from build123d import *

# Parameters (mm, degrees)
EXTRUDE_1_DEPTH     = 22.5
SKETCH_2_R          = 11
CUT_EXTRUDE_2_DEPTH = 18
CUT_EXTRUDE_3_REACH = 24.5
SKETCH_3_R          = 4
CHAMFER_1_SIZE      = 1


with BuildPart() as part:
    # Эскиз1 → Бобышка-Вытянуть1 (new body)
    with BuildSketch(Plane(origin=(0, 0, 0), x_dir=(1, 0, 0), z_dir=(0, 1, 0))):
        Polygon((17.320508076, 0), (8.660254038, 15), (-8.660254038, 15), (-17.320508076, 0), (-8.660254038, -15), (8.660254038, -15), align=None)
    extrude(amount=EXTRUDE_1_DEPTH)

    # Эскиз2 → Вырез-Вытянуть2 (cut)
    with BuildSketch(Plane(origin=(0, 22.5, 0), x_dir=(1, 0, 0), z_dir=(0, 1, 0))):
        Circle(SKETCH_2_R)
    extrude(amount=-CUT_EXTRUDE_2_DEPTH, mode=Mode.SUBTRACT)

    # Эскиз3 → Вырез-Вытянуть3 (cut, up to next)
    with BuildSketch(Plane.XZ, mode=Mode.PRIVATE) as cut_extrude_3_sk1:
        Circle(SKETCH_3_R)
    cut_extrude_3_tool1 = extrude(cut_extrude_3_sk1.sketch, amount=-CUT_EXTRUDE_3_REACH, mode=Mode.PRIVATE) & part.part
    add(cut_extrude_3_tool1.solids().sort_by_distance((0, 0, 0))[0], mode=Mode.SUBTRACT)

    # Эскиз4 → Вырез-Повернуть1 (revolve, cut)
    with BuildSketch(Plane(origin=(0, 0, 0), x_dir=(-0.5, 0, 0.866025404), z_dir=(-0.866025404, 0, -0.5))):
        Polygon((-17.320508076, 18.345818937), (-17.320508076, 22.5), (-14.628303654, 22.5), align=None)
    cut_revolve_1 = revolve(axis=Axis((0, 0, 0), (0, 1, 0)), mode=Mode.SUBTRACT)

    # Зеркальное отражение1: Вырез-Повернуть1 across plane
    add(cut_revolve_1.mirror(Plane.ZX.offset(11.25)), mode=Mode.SUBTRACT)

    # Фаска1
    chamfer_1_edges = [part.edges().sort_by_distance(p)[0] for p in [
        (-11, 22.5, 0),
    ]]
    chamfer(chamfer_1_edges, length=CHAMFER_1_SIZE)


solid = part.part
Design review of the part built by this model. Coordinates are the model's own, in mm. A direction names the side the tool comes from. Coordinates: 2 decimals unless noted, no trailing zeros. Loops run counter-clockwise (first coordinate to the right, second up) from the corner with the lowest first, then second, coordinate; pieces in that order, holes last.
Item 1: Clearance check with flat-ended pins moving along their axes: pin 1 (10 mm diameter, centred on x = 6.5, z = -0.5, fed in from -Y); pin 2 (1.5 mm diameter, centred on y = 7.5, z = 5, fed in from -X); pin 3 (1 mm diameter, centred on y = 5, z = 6.5, fed in from -X); pin 4 (17.5 mm diameter, centred on x = 0, z = 0, fed in from +Y). State where each tip first meets the part, or that it passes through.
Completed:
pin 1: stops at y = 0
pin 2: stops at x = -14.87
pin 3: stops at x = -13.86
pin 4: stops at y = 4.5
Item 2: For faces 1 (the flat face through (0, 11, -15)), 2 (the flat face through (0, 4.5, 5)), list the 3-axis set-ups (+Z, -Z, +X, -X, +Y, -Y) from which the entire face can be reached by the end or side of a thin tool; tool diameter is ignored.
Completed:
face 1: -Z, +X, -X, +Y, -Y
face 2: +Y
Item 3: Add section B-B (y = 16.75). Write out the cut boundary in (x, z).
Completed:
outline: (-17.32, 0) - (-8.66, -15) - (8.66, -15) - (17.32, 0) - (8.66, 15) - (-8.66, 15) - close; hole circle Ø22 at (0, 0)
Item 4: Add section A-A (x = 0). Write out the cut boundary in (y, z).
Completed:
outline: (0, -14.63) - (0.57, -15) - (21.93, -15) - (22.5, -14.63) - (22.5, -12) - (21.5, -11) - (4.5, -11) - (4.5, -4) - (0, -4) - close; (0, 4) - (4.5, 4) - (4.5, 11) - (21.5, 11) - (22.5, 12) - (22.5, 14.63) - (21.93, 15) - (0.57, 15) - (0, 14.63) - close
Item 5: Wall thickness on L1, parallel to Z at x = 0, y = 2.65; L2, parallel to Z at x = 0, y = 11; L3, parallel to X at y = 10.75, z = -10: over which ranges is each line inside the solid? List them lowest first.
Completed:
L1: z = -15 to -4, 4 to 15
L2: z = -15 to -11, 11 to 15
L3: x = -11.55 to -4.58, 4.58 to 11.55
Item 6: Draft analysis for pull direction Z (two halves, no side actions). For faces 3 (the cylindrical face through (-0.867, 2.218, -3.905)), 4 (the cylindrical face through (-2.38, 13.12, 10.74)), 5 (the flat face through (13.05, 11.1, -7.4)), 6 (the flat face through (0, 11, 15)), state which applies: pulls with the +Z half, pulls with the -Z half, needs draft (parallel to the pull), parting line crosses it, or undercut.
Completed:
face 3: undercut
face 4: undercut
face 5: pulls with the -Z half
face 6: pulls with the +Z half
Item 7: Add section C-C (y = 19.75). Write out the cut boundary in (x, z).
Completed:
outline: (-16.32, -1.74) - (-9.66, -13.26) arc R16.41 ccw to (-6.66, -15) - (6.66, -15) arc R16.41 ccw to (9.66, -13.26) - (16.32, -1.74) arc R16.41 ccw to (16.32, 1.74) - (9.66, 13.26) arc R16.41 ccw to (6.66, 15) - (-6.66, 15) arc R16.41 ccw to (-9.66, 13.26) - (-16.32, 1.74) arc R16.41 ccw to start; hole circle Ø22 at (0, 0)
